Geometry: final body of the model. Coordinates: model frame, mm. Face numbers are marked on the shaded views. A direction names the side the tool comes from. Give positions to 0.01 mm unless a question says otherwise; leave off trailing zeros. Loops run counter-clockwise (first coordinate to the right, second up) from the corner with the lowest first, then second, coordinate; pieces in that order, holes last. Notation, with made-up numbers: (-17, 82) - (36, 82) arc R26 ccw to (36, 101) - close; hole circle Ø6 at (14, -14.75). An arc over 180 degrees is marked (long way). Answer in a Markdown table with one row per item.
from build123d import *

# Parameters (mm, degrees)
F0_W     = 177.8
F0_H     = 76.2
F1_DEPTH = 50.8
F2_T     = -2.54
F4_DEPTH = 76.201
F6_DEPTH = 76.201
F8_DEPTH = 76.201


with BuildPart() as f1:
    # F0 (on Top) → F1 (new body)
    with BuildSketch(Plane.XY):
        with Locations((23.041371, -18.925695)):
            Rectangle(F0_W, F0_H)
    extrude(amount=F1_DEPTH)

    # F2
    f2_openings = [f1.faces().sort_by_distance(p)[0] for p in [
        (23.041371, -18.925695, 50.8),
        (-65.858629, -18.925695, 25.4),
        (111.941371, -18.925695, 25.4),
    ]]
    offset(amount=F2_T, openings=f2_openings)

    # F3 (on face) → F4 (cut, through all)
    with BuildSketch(Plane.XZ.offset(57.025695)):
        Polygon((-74.445255, 69.43772), (-65.858629, 0), (-48.242956, 50.8), (-10.39157, 50.8), (11.275085, 22.44979), (25.632508, 50.8), (59.82928, 50.8), (111.941371, 0), (111.941371, 69.43772), align=None)
    extrude(amount=-F4_DEPTH, mode=Mode.SUBTRACT)

    # F5 (on face) → F6 (cut, through all)
    with BuildSketch(Plane.XZ.offset(57.025695)):
        Polygon((-41.716851, 36.807209), (-47.720864, 16.18473), (0, 15.662642), (-13.263052, 36.807209), align=None)
    extrude(amount=-F6_DEPTH, mode=Mode.SUBTRACT)

    # F7 (on face) → F8 (cut, through all)
    with BuildSketch(Plane.XZ.offset(57.025695)):
        Polygon((31.897567, 39.156608), (19.889543, 15.140554), (69.74896, 15.140554), (53.82527, 39.156608), align=None)
    extrude(amount=-F8_DEPTH, mode=Mode.SUBTRACT)


solid = f1.part
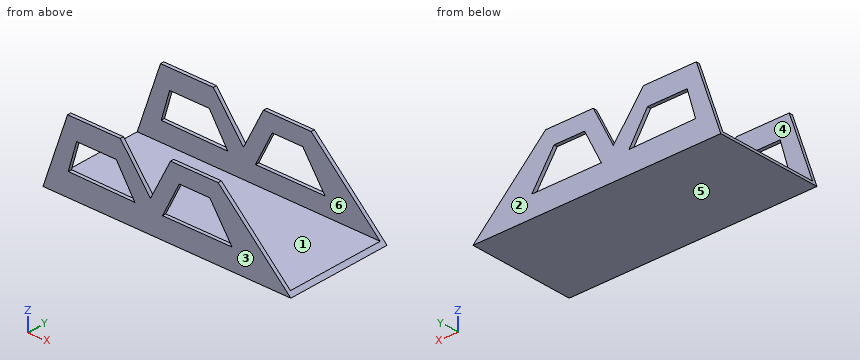
Q1. First-contact query: pin 1 (2 mm diameter, centred on x = 10, y = 10, fed in from +Z). Flat tip, straight axial feed; report the tip coordinate or a pass-through.
Check values:
| item | result |
|---|---|
| pin 1 | z = 2.54 |
Q2. Material intervals for line 1 along Y through (x, z) = (88, 13); line 2 along Z through (x, y) = (-55, -29), sorted ascending.
Check values:
| item | result |
|---|---|
| line 1 | -57.03 to -54.49, 16.63 to 19.17 |
| line 2 | 0 to 2.54 |
Q3. Draft query along Y for the marked faces 1, 2, 3 and 4. Return one class per face: pulls with the +Y half, pulls with the -Y half, needs draft (parallel to the pull), parting line crosses it, or undercut.
Check values:
| item | result |
|---|---|
| face 1 | undercut |
| face 2 | pulls with the +Y half |
| face 3 | pulls with the -Y half |
| face 4 | undercut |
Q4. Cut plane A-A (z = 20). Output: boundary loops of the cut face in (x, y), and give its area (3 significant figures).
Check values:
| item | result |
|---|---|
| outline | (-58.92, -57.03) - (-46.61, -57.03) - (-46.61, -54.49) - (-58.92, -54.49) - close; (-58.92, 16.63) - (-46.61, 16.63) - (-46.61, 19.17) - (-58.92, 19.17) - close; (-2.72, -57.03) - (22.32, -57.03) - (22.32, -54.49) - (-2.72, -54.49) - close; (-2.72, 16.63) - (22.32, 16.63) - (22.32, 19.17) - (-2.72, 19.17) - close; (66.53, -57.03) - (91.42, -57.03) - (91.42, -54.49) - (66.53, -54.49) - close; (66.53, 16.63) - (91.42, 16.63) - (91.42, 19.17) - (66.53, 19.17) - close |
| area | 316 mm² |
Q5. Cut plane D-D (z = 31.5). Give the number of separate pieces and of enclosed holes in the cut face, and give its area (3 significant figures).
Check values:
| item | result |
|---|---|
| separate pieces | 8 |
| enclosed holes | 0 |
| area | 299 mm² |
Q6. Cut plane B-B (x = 40.5). Output: boundary loops of the cut face in (y, z), and give its area (3 significant figures).
Check values:
| item | result |
|---|---|
| outline | (-57.03, 0) - (19.17, 0) - (19.17, 15.14) - (16.63, 15.14) - (16.63, 2.54) - (-54.49, 2.54) - (-54.49, 15.14) - (-57.03, 15.14) - close; (-57.03, 39.16) - (-54.49, 39.16) - (-54.49, 50.8) - (-57.03, 50.8) - close; (16.63, 39.16) - (19.17, 39.16) - (19.17, 50.8) - (16.63, 50.8) - close |
| area | 317 mm² |
Q7. Reachability of the marked faces 5 and 6 from +Z, -Z, +X, -X, +Y, -Y: full face, straight path, thin tool, end or side. Return the list, or none.
Check values:
| item | result |
|---|---|
| face 5 | -Z, +X, -X, +Y, -Y |
| face 6 | +Z, +X, -X |
Q8. Cut plane C-C (z = 7). Output: boundary loops of the cut face in (x, y), and give its area (3 significant figures).
Check values:
| item | result |
|---|---|
| outline | (-63.43, -57.03) - (104.76, -57.03) - (104.76, -54.49) - (-63.43, -54.49) - close; (-63.43, 16.63) - (104.76, 16.63) - (104.76, 19.17) - (-63.43, 19.17) - close |
| area | 854 mm² |
